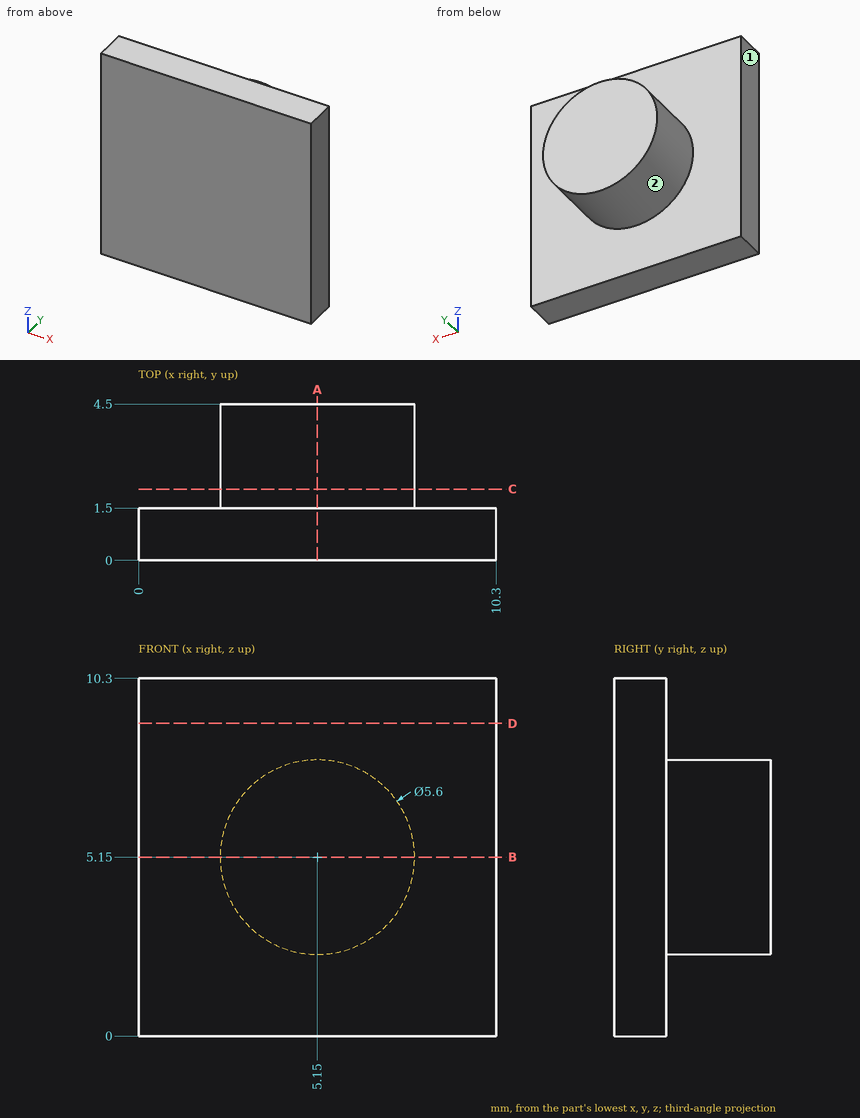
Geometry: see drawing. Coordinates: mm, zero at the bounding-box minimum. A direction names the side the tool comes from. Give positions to 0.01 mm unless a question says otherwise; leave off trailing zeros. Order: outer loops, then holes, each group sorted by start corner. A loop starts at its lowest first (then second) coordinate and runs counter-clockwise, first axis right, second up. Notation, with made-up numbers: M 11.5,74 L 21.5,74 A27 ccw 21.5,105 Z; hole C -3.5,41.5 d9. An arc over 180 degrees is marked long. Answer as a JSON object with one key per item and string values.
1. Cut plane C-C, the plane y = 2.05. Output: boundary loops of the cut face in (x, z), and give its area (3 significant figures).
Result sheet:
{"outline": "C 5.15,5.15 d5.6", "area": "24.6 mm²"}
2. Reachability of the marked faces 1 and 2 from +Z, -Z, +X, -X, +Y, -Y: full face, straight path, thin tool, end or side. Return the list, or none.
Result sheet:
{"face 1": "+Z, -Z, -X, +Y, -Y", "face 2": "+Y"}
3. Ray query, line 1 (Y direction, x = 9.5, z = 9.75); line 2 (Z direction, x = 6.75, y = 3.1); line 3 (X direction, y = 3.75, z = 5.5). Return the intervals inside material, ascending. Write a range as [from, to].
Result sheet:
{"line 1": "[0, 1.5]", "line 2": "[2.85, 7.45]", "line 3": "[2.37, 7.93]"}
4. Cut plane A-A, the plane x = 5.15. Output: boundary loops of the cut face in (y, z), and give its area (4 significant figures).
Result sheet:
{"outline": "M 0,0 L 1.5,0 L 1.5,2.35 L 4.5,2.35 L 4.5,7.95 L 1.5,7.95 L 1.5,10.3 L 0,10.3 Z", "area": "32.25 mm²"}
5. Cut plane D-D, the plane z = 9. Output: boundary loops of the cut face in (x, y), and give its area (4 significant figures).
Result sheet:
{"outline": "M 0,0 L 10.3,0 L 10.3,1.5 L 0,1.5 Z", "area": "15.45 mm²"}
6. Cut plane B-B, the plane z = 5.15. Output: boundary loops of the cut face in (x, y).
Result sheet:
{"outline": "M 0,0 L 10.3,0 L 10.3,1.5 L 7.95,1.5 L 7.95,4.5 L 2.35,4.5 L 2.35,1.5 L 0,1.5 Z"}
